from build123d import *

# Parameters (mm, degrees)
F0_W     = 80
F0_H     = 40
F1_DEPTH = 60
F2_R     = 15
F3_DEPTH = 40.001


with BuildPart() as f1:
    # F0 (on Front) → F1 (new body)
    with BuildSketch(Plane.XZ):
        Rectangle(F0_W, F0_H)
    extrude(amount=F1_DEPTH)

    # F2 (on face) → F3 (cut, through all)
    with BuildSketch(Plane.XY.offset(20)):
        with Locations((0, -28.49043)):
            Circle(F2_R)
    extrude(amount=-F3_DEPTH, mode=Mode.SUBTRACT)


solid = f1.part
Read the model definition and answer for the solid it produces. Units are mm, in the model's axes. Round coordinates to 2 decimals unless told otherwise and drop trailing zeros. Order: outer loops, then holes, each group sorted by start corner. A loop starts at its lowest first (then second) coordinate and runs counter-clockwise, first axis right, second up.
1) A flat-ended cylindrical pin translates along its axis: pin 1 (18 mm diameter, centred on x = 0, y = -28.49, fed in from -Z). Find the tip coordinate at first contact, or state that the pin passes through.
2) The part is cut by section B-B on z = -17.5. Write down the section's boundary in (x, y), plus the area to 3 significant figures.
3) Straight lines are drawn through the part: L1, parallel to Y at x = 0, z = 1.5; L2, parallel to X at y = -23.5, z = 13; L3, parallel to X at y = -15.5, z = -7. For each, find the intervals that lie inside material, in ascending order.
4) The mould has two halves that part along X. Classify faces 1 (the face through (-1.953, -13.618, 0.28)), 2 (the face through (-40, -30, 0)), 3 (the face through (-9, -43, -20)): released by +X, released by -X, zero draft, split by the parting line, or undercut.
5) The part is cut by section A-A on x = 0. Write down the section's boundary in (y, z), plus the area to 3 significant figures.
Resolved:
1. pin 1: passes through
2. outline: (-40, -60) - (40, -60) - (40, 0) - (-40, 0) - close; hole circle Ø30 at (0, -28.49)
2. area: 4,090 mm2
3. L1: y = -60 to -43.49, -13.49 to 0
3. L2: x = -40 to -14.15, 14.15 to 40
3. L3: x = -40 to -7.5, 7.5 to 40
4. face 1: undercut
4. face 2: released by -X
4. face 3: zero draft
5. outline: (-60, -20) - (-43.49, -20) - (-43.49, 20) - (-60, 20) - close; (-13.49, -20) - (0, -20) - (0, 20) - (-13.49, 20) - close
5. area: 1,200 mm2
